from build123d import *

# Parameters (mm, degrees)
SKETCH1_R           = 35
BOSS_EXTRUDE1_DEPTH = 35
SKETCH2_R           = 40
BOSS_EXTRUDE2_DEPTH = 10
SKETCH3_R           = 2
CUT_EXTRUDE1_DEPTH  = 10
CIRPATTERN1_COUNT   = 6


with BuildPart() as part:
    # Sketch1 → Boss-Extrude1 (new body)
    with BuildSketch(Plane(origin=(0, 0, 0), x_dir=(0, 0, -1), z_dir=(1, 0, 0))):
        Circle(SKETCH1_R)
    extrude(amount=BOSS_EXTRUDE1_DEPTH)

    # Sketch2 → Boss-Extrude2 (add)
    with BuildSketch(Plane(origin=(35, 0, 0), x_dir=(0, 0, -1), z_dir=(1, 0, 0))):
        Circle(SKETCH2_R)
    extrude(amount=BOSS_EXTRUDE2_DEPTH)

    # Sketch3 → Cut-Extrude1 (cut)
    with BuildSketch(Plane(origin=(0, 35, 0), x_dir=(1, 0, 0), z_dir=(0, 1, 0))):
        with Locations((15, 0)):
            Circle(SKETCH3_R)
    cut_extrude1 = extrude(amount=-CUT_EXTRUDE1_DEPTH, mode=Mode.SUBTRACT)

    # CirPattern1: Cut-Extrude1 ×6 about axis
    cirpattern1_axis = Axis((0, 0, 0), (1, 0, 0))
    for i in range(1, CIRPATTERN1_COUNT):
        add(cut_extrude1.rotate(cirpattern1_axis, i * 360 / CIRPATTERN1_COUNT), mode=Mode.SUBTRACT)


solid = part.part
Could you check a few things on this model? Use its own coordinates, in mm. A direction names the side the tool comes from. Round coordinates to 2 decimals unless told otherwise and drop trailing zeros. Order: outer loops, then holes, each group sorted by start corner. A loop starts at its lowest first (then second) coordinate and runs counter-clockwise, first axis right, second up. Notation, with made-up numbers: M 88,-27 L 127,-27 A27 ccw 127,0 Z; hole C -16,18.5 d9. An arc over 180 degrees is marked long. One line per item, written item: value.
(1) Imagine slicing it at C-C (x = 15). Write out the boundary of the cut face in (y, z).
Ans:
outline: M -34.94,-2 A35 ccw -19.2,-29.26 L -14.23,-20.65 L -10.77,-22.65 L -15.74,-31.26 A35 ccw 15.74,-31.26 L 10.77,-22.65 L 14.23,-20.65 L 19.2,-29.26 A35 ccw 34.94,-2 L 25,-2 L 25,2 L 34.94,2 A35 ccw 19.2,29.26 L 14.23,20.65 L 10.77,22.65 L 15.74,31.26 A35 ccw -15.74,31.26 L -10.77,22.65 L -14.23,20.65 L -19.2,29.26 A35 ccw -34.94,2 L -25,2 L -25,-2 Z
(2) Which directions (+Z, -Z, +X, -X, +Y, -Y) give clear straight access to the entire face, cutting with the end or side of a thin tool? Please do faces 5 (the cylindrical face through (13.4, 30.1, 1.2)), 6 (the cylindrical face through (17, -21, 28)), 7 (the flat face through (14.97, -12.52, -21.64)), 8 (the flat face through (15, -25, 0)).
Ans:
face 5: +Y
face 6: -X
face 7: none
face 8: -Y
(3) I'm going to push flat-ended pins straight in: P1, Ø3, axis at x = 6, z = 26, coming from the +Y side (3 decimals); P2, Ø1.5, axis at x = 33, y = -23.5, coming from the -Z side; P3, Ø1, axis at x = 12.5, y = -6.5, coming from the -Z side; P4, Ø24, axis at y = -9.5, z = -15.5, coming from the -X side. Where does each tip first touch, or does it pass through?
Ans:
P1: stops at y = 24.995
P2: stops at z = -26.6
P3: stops at z = -34.48
P4: stops at x = 0
(4) I need wall thicknesses on line 1 along X through (y, z) = (27.75, 0); line 2 along X through (y, z) = (-16.5, 34); line 3 along Y through (x, z) = (22.5, -0.5). Which ranges of each line are inside material? Lowest first, please. Write a range as from..to.
Ans:
line 1: x = 0..13, 17..45
line 2: x = 35..45
line 3: y = -35..35
(5) Imagine slicing it at A-A (z = 0). Write out the boundary of the cut face in (x, y).
Ans:
outline: M 0,-35 L 13,-35 L 13,-25 L 17,-25 L 17,-35 L 35,-35 L 35,-40 L 45,-40 L 45,40 L 35,40 L 35,35 L 17,35 L 17,25 L 13,25 L 13,35 L 0,35 Z
(6) If we mould it in two halves opening along Y, with no side actions, what happens to faces 1 (the flat face through (15, 25, 0)), 2 (the flat face through (14.97, 12.48, -21.66)), 3 (the cylindrical face through (13.53, 13.86, -26.72)), 4 (the flat face through (35, -35.4, 0.2))? For each: released by +Y, released by -Y, zero draft, split by the parting line, or undercut.
Ans:
face 1: released by +Y
face 2: undercut
face 3: undercut
face 4: zero draft
(7) Imagine slicing it at D-D (z = -24.5). Count the separate pieces of the cut face and the enclosed holes in it, and give its area (3 significant figures).
Ans:
separate pieces: 1
enclosed holes: 2
area: 2,350 mm^2
(8) Imagine slicing it at B-B (y = 0). Write out the boundary of the cut face in (x, z).
Ans:
outline: M 0,-35 L 35,-35 L 35,-40 L 45,-40 L 45,40 L 35,40 L 35,35 L 0,35 Z
